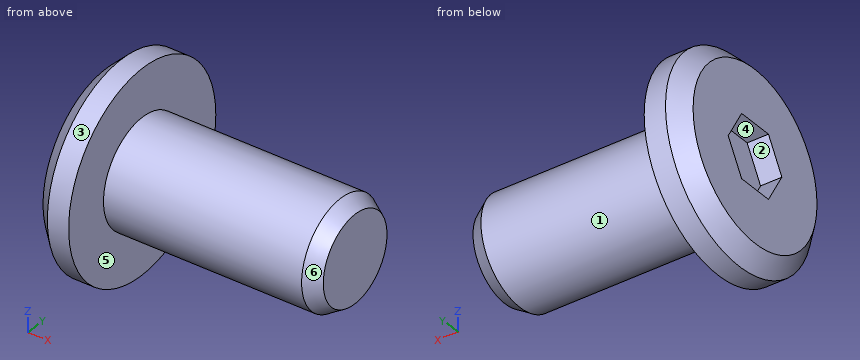
from build123d import *

# Parameters (mm, degrees)
CUT_EXTRUDE1_DEPTH = 1
CHAMFER1_SIZE      = 0.75


with BuildPart() as part:
    # Sketch1 → Revolve1 (revolve)
    with BuildSketch(Plane.XY):
        Polygon((11.75, 0), (11.75, 2.057236169), (11.055, 2.5), (1.75, 2.5), (1.75, 4.75), (0, 4.75), (0, 0), align=None)
    revolve(axis=Axis((0, 0, 0), (1, 0, 0)))

    # Sketch5 → Cut-Extrude1 (cut)
    with BuildSketch(Plane.ZY):
        Polygon((1.5, -0.866025404), (1.5, 0.866025404), (0, 1.732050808), (-1.5, 0.866025404), (-1.5, -0.866025404), (0, -1.732050808), align=None)
    extrude(amount=-CUT_EXTRUDE1_DEPTH, mode=Mode.SUBTRACT)

    # Chamfer1
    chamfer1_edges = [part.edges().sort_by_distance(p)[0] for p in [
        (0, -4.75, 0),
    ]]
    chamfer(chamfer1_edges, length=CHAMFER1_SIZE)


solid = part.part
Could you check a few things on this model? Use its own coordinates, in mm. Face numbers are marked on the shaded views. A direction names the side the tool comes from. Round coordinates to 2 decimals unless told otherwise and drop trailing zeros. Loops run counter-clockwise (first coordinate to the right, second up) from the corner with the lowest first, then second, coordinate; pieces in that order, holes last. Notation, with made-up numbers: (35.25, 70.25) - (87.25, 70.25) arc R26 ccw to (87.25, 101.25) - close; hole circle Ø7 at (30.5, 88). An arc over 180 degrees is marked (long way). Write item = value, one per line.
1) I need wall thicknesses on line 1 along X through (y, z) = (1.25, 0.5); line 2 along X through (y, z) = (-0.75, 3.25); line 3 along Y through (x, z) = (6, -2). Which ranges of each line are inside material? Lowest first, please. Write a range as from..to.
Computed:
line_1 = 1..11.75
line_2 = 0..1.75
line_3 = -1.5..1.5
2) If we mould it in two halves opening along Y, with no side actions, what happens to the marked faces 4, 5 and 6? For each: pulls with the +Y half, pulls with the -Y half, needs draft (parallel to the pull), parting line crosses it, or undercut.
Computed:
face_4 = undercut
face_5 = needs draft
face_6 = parting line crosses it
3) Imagine slicing it at A-A (y = 0). Please give me the cut outline in (x, z) (3 decimals).
Computed:
outline = (0, -4) - (0.75, -4.75) - (1.75, -4.75) - (1.75, -2.5) - (11.055, -2.5) - (11.75, -2.057) - (11.75, 2.057) - (11.055, 2.5) - (1.75, 2.5) - (1.75, 4.75) - (0.75, 4.75) - (0, 4) - (0, 1.5) - (1, 1.5) - (1, -1.5) - (0, -1.5) - close
4) I'm going to push flat-ended pins straight in: P1, Ø3, axis at x = 6.5, z = -2.5, coming from the -Y side; P2, Ø1.1, axis at x = 0.5, y = 0, coming from the +Z side; P3, Ø4, axis at x = 10, y = 0.5, coming from the +Z side; P4, Ø1.5, axis at y = -0.5, z = -0.5, coming from the -X side. Where does each tip first touch, or does it pass through?
Computed:
P1 = -2.29
P2 = 4.75
P3 = 2.5
P4 = 1
5) Imagine slicing it at B-B (x = 10). Please give me the cut outline in (y, z).
Computed:
outline = circle Ø5 at (0, 0)
6) On a 3-axis mill with a long thin cutter (end or side, diameter ignored), from which of +Z, -Z, +X, -X, +Y, -Y can I reach the whole of each face in a straight line? I mean the marked faces 1, 2 and 3. Say none if no direction works.
Computed:
face_1 = +X
face_2 = -X
face_3 = +X, -X
7) Imagine slicing it at C-C (x = 11.25). Please give me the cut outline in (y, z).
Computed:
outline = circle Ø4.75 at (0, 0)
